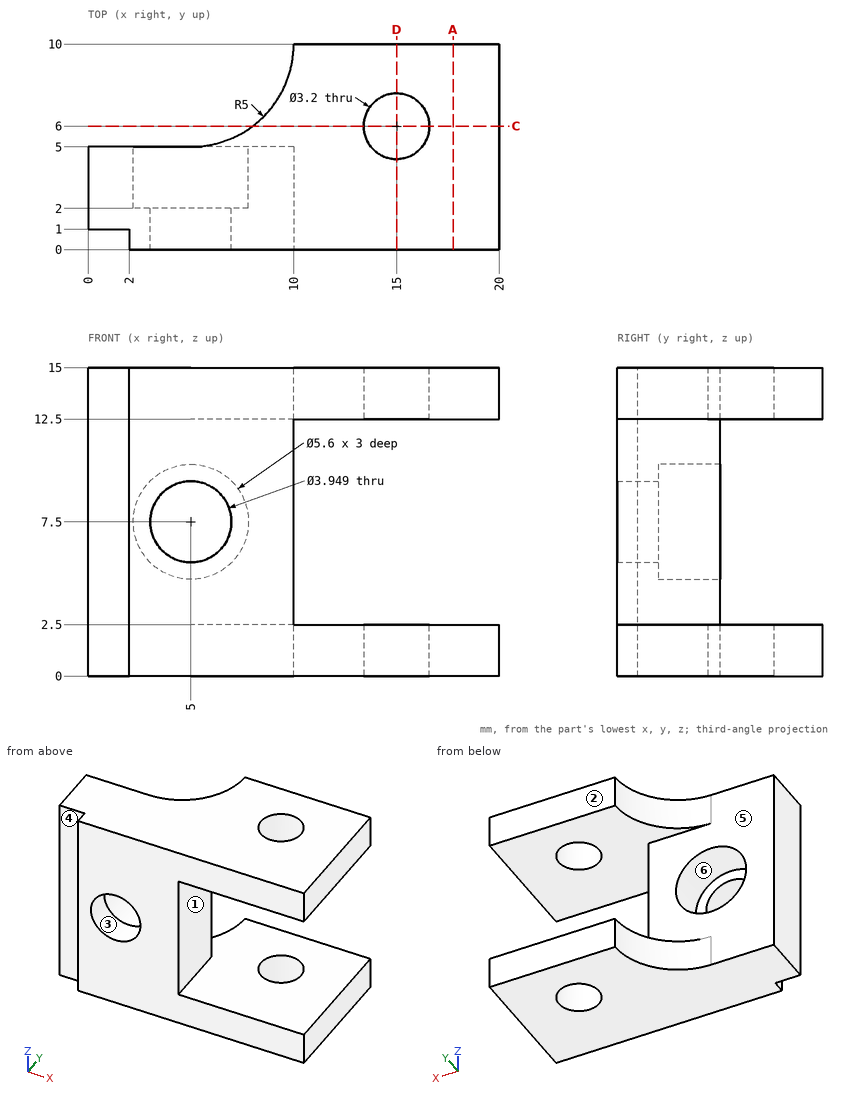
Drawing for the job (mm, zero at the part's lowest x, y, z). A direction names the side the tool comes from. Coordinates: 2 decimals unless noted, no trailing zeros. Order: outer loops, then holes, each group sorted by start corner. A loop starts at its lowest first (then second) coordinate and runs counter-clockwise, first axis right, second up. Notation, with made-up numbers: (10, 88) - (65, 88) arc R21 cw to (65, 92) - close; hole circle Ø9 at (27.5, -29). An arc over 180 degrees is marked (long way). Use a Markdown table: item, result. Add a question column.
(1) Saw through at D-D (x = 15). Give the cut face in (y, z).
(2) Saw through at A-A (x = 17.75). Give the cut face in (y, z).
(3) Saw through at C-C (y = 6). Give the cut face in (x, z), then the cut area to 3 significant figures.
(4) Pull direction X, two halves, no side cores. Call the marked faces 1, 2 and 3: +X half, -X half, draft (parallel to the pull), parting line (faces both ways), or undercut.
(5) Drill centre lines: line 1 along Z through (x, y) = (16.5, 4.25); line 2 along X through (y, z) = (0.75, 7.5); line 3 along X through (y, z) = (3.95, 7.5). Where is each one in solid material? Low to high. Write a range as [from, to].
(6) Flat gauge pins, fed straight in: pin 1 (1.1 mm diameter, centred on y = 0.5, z = 4.5, fed in from -X); pin 2 (4.5 mm diameter, centred on x = 5, z = 7.5, fed in from +Y); pin 3 (6.5 mm diameter, centred on x = 5, z = 7.5, fed in from +Y); pin 4 (6 mm diameter, centred on y = 8.5, z = 2.5, fed in from -X). Where does each tip first touch, or does it go through?
(7) Which spindle directions (+Z, -Z, +X, -X, +Y, -Y) get a long thin tool onto all of the face, cutting with end or side? Do the marked faces 4, 5 and 6. Say none if no direction does.
Solved:
| question | item | result |
|---|---|---|
| 1 | outline | (0, 0) - (4.4, 0) - (4.4, 2.5) - (0, 2.5) - close; (0, 12.5) - (4.4, 12.5) - (4.4, 15) - (0, 15) - close; (7.6, 0) - (10, 0) - (10, 2.5) - (7.6, 2.5) - close; (7.6, 12.5) - (10, 12.5) - (10, 15) - (7.6, 15) - close |
| 2 | outline | (0, 0) - (10, 0) - (10, 2.5) - (0, 2.5) - close; (0, 12.5) - (10, 12.5) - (10, 15) - (0, 15) - close |
| 3 | outline | (8, 0) - (13.4, 0) - (13.4, 2.5) - (8, 2.5) - close; (8, 12.5) - (13.4, 12.5) - (13.4, 15) - (8, 15) - close; (16.6, 0) - (20, 0) - (20, 2.5) - (16.6, 2.5) - close; (16.6, 12.5) - (20, 12.5) - (20, 15) - (16.6, 15) - close |
| 3 | area | 44.0 mm² |
| 4 | face 1 | +X half |
| 4 | face 2 | draft |
| 4 | face 3 | undercut |
| 5 | line 1 | z = [0, 2.5], [12.5, 15] |
| 5 | line 2 | x = [2, 3.03], [6.97, 10] |
| 5 | line 3 | x = [0, 2.2], [7.8, 10] |
| 6 | pin 1 | stops at x = 0 |
| 6 | pin 2 | stops at y = 2 |
| 6 | pin 3 | stops at y = 5 |
| 6 | pin 4 | stops at x = 7.18 |
| 7 | face 4 | +Z, -Z, -X, -Y |
| 7 | face 5 | -X, +Y |
| 7 | face 6 | +Y |
